Part model, mm, in its own coordinate system. A direction names the side the tool comes from. Round coordinates to 2 decimals unless told otherwise and drop trailing zeros. Order: outer loops, then holes, each group sorted by start corner. A loop starts at its lowest first (then second) coordinate and runs counter-clockwise, first axis right, second up. Notation, with made-up numbers: M 39,34 L 91,34 A19 ccw 91,43 Z; hole C 85,63 d7. An arc over 180 degrees is marked long. One line per question, with ' | ' between items.
from build123d import *

# Parameters (mm, degrees)
BOSS_EXTRUDE1_DEPTH     = 12.7
CUT_EXTRUDE1_REACH      = 14.7
SKETCH2_R               = 0.775
SKETCH4_R               = 12.5
SKETCH4_R_2             = 2.75
BOSS_EXTRUDE3_DEPTH     = 20.5
BOSS_EXTRUDE4_DEPTH     = 20.5
SKETCH5_R               = 1.5
CUT_EXTRUDE2_DEPTH      = 12
CUT_EXTRUDE2_DEPTH_BACK = 2
CUT_EXTRUDE3_DEPTH      = 17


with BuildPart() as part:
    # Sketch1 → Boss-Extrude1 (new body)
    with BuildSketch(Plane(origin=(0, 0, 0), x_dir=(-1, 0, 0), z_dir=(0, 0, -1))):
        Polygon((22.52557458, -1.736588639), (22.52557458, 0.194536921), (19.229808022, 0.93665661), (15.128723263, 11.851737372), (17.063649078, 14.621011813), (15.786423571, 16.069438867), (12.890863827, 14.329165151), (2.313040546, 19.235032954), (1.719665356, 22.560799741), (-0.211460204, 22.560799741), (-0.98374926, 19.271971918), (-11.902473648, 15.180597821), (-14.673902719, 17.112436257), (-16.073066924, 15.781427071), (-14.308800518, 12.900423272), (-19.236913758, 2.332945609), (-22.560976284, 1.730096406), (-22.560976284, -0.201029153), (-19.275488766, -0.987407309), (-15.174404006, -11.902488071), (-17.112216048, -14.669743631), (-15.788139908, -16.075470597), (-12.910837913, -14.305173427), (-2.333014633, -19.21104123), (-1.727718406, -22.534659035), (0.203407153, -22.534659035), (0.978499423, -19.246490729), (11.89722381, -15.155116632), (14.659649692, -17.099807376), (16.072878525, -15.783741196), (14.276312796, -12.922767512), (19.204426036, -2.355289849), align=None)
    extrude(amount=-BOSS_EXTRUDE1_DEPTH)

    # Sketch2 → Cut-Extrude1 (cut, up to next)
    with BuildSketch(Plane(origin=(0, 0, 0), x_dir=(-1, 0, 0), z_dir=(0, 0, -1)), mode=Mode.PRIVATE) as cut_extrude1_sk1:
        with Locations((-0.019773646, -0.00956531)):
            Circle(SKETCH2_R)
    cut_extrude1_tool1 = extrude(cut_extrude1_sk1.sketch, amount=-CUT_EXTRUDE1_REACH, mode=Mode.PRIVATE) & part.part
    add(cut_extrude1_tool1.solids().sort_by_distance((0.019774, -0.009565, 0))[0], mode=Mode.SUBTRACT)

    # Sketch4 → Boss-Extrude3 (add)
    with BuildSketch(Plane(origin=(0, 0, 0), x_dir=(-1, 0, 0), z_dir=(0, 0, -1))):
        Circle(SKETCH4_R)
        Circle(SKETCH4_R_2, mode=Mode.SUBTRACT)
    extrude(amount=BOSS_EXTRUDE3_DEPTH)

    # Sketch4<4> → Boss-Extrude4 (add)
    with BuildSketch(Plane(origin=(0, 0, 0), x_dir=(-1, 0, 0), z_dir=(0, 0, -1))):
        with BuildLine():
            Line((-0.567488363, 2.690809722), (0.726565511, 2.652282518))
            ThreePointArc((0.726565511, 2.652282518), (0.081838079, 2.748782008), (-0.567488363, 2.690809722))
        make_face()
    extrude(amount=BOSS_EXTRUDE4_DEPTH)

    # Sketch5 → Cut-Extrude2 (cut, two sides)
    with BuildSketch(Plane(origin=(0, 4, 0), x_dir=(1, 0, 0), z_dir=(0, 1, 0))) as cut_extrude2_sk:
        with Locations((0, 16.130068411)):
            Circle(SKETCH5_R)
    extrude(amount=CUT_EXTRUDE2_DEPTH, mode=Mode.SUBTRACT)
    extrude(cut_extrude2_sk.sketch, amount=-CUT_EXTRUDE2_DEPTH_BACK, mode=Mode.SUBTRACT)

    # Sketch6 → Cut-Extrude3 (cut)
    with BuildSketch(Plane(origin=(0, 0, -20.5), x_dir=(-1, 0, 0), z_dir=(0, 0, -1))):
        Polygon((4.579538574, 7.537569925), (-4.420461426, 7.805522315), (-4.538346431, 3.845994095), (4.461653569, 3.578041705), align=None)
    extrude(amount=-CUT_EXTRUDE3_DEPTH, mode=Mode.SUBTRACT)


solid = part.part
1) Saw through at A-A (z = -5). List the corners of the cut face in (x, y).
The answers:
outline: C 0,0 d25; hole M -4.58,7.54 L -4.46,3.58 L 4.54,3.85 L 4.42,7.81 Z; hole M -0.73,2.65 A2.75 ccw long 0.57,2.69 Z
2) Which spindle directions (+Z, -Z, +X, -X, +Y, -Y) get a long thin tool onto all of the face, cutting with end or side? Do faces 1 (the face through (6.367, 17.255, 6.261)), 2 (the face through (1.43, 3.04, -16.58)), 3 (the face through (14.37, -15.203, 6.261)), 4 (the face through (-16.083, 13.217, 6.261)), 5 (the face through (0, 6, -3.5)). Say none if no direction does.
The answers:
face 1: +Z, -Z, +Y | face 2: +Y | face 3: +Z, -Z, -Y | face 4: +Z, -Z, -X | face 5: -Z
3) Drop flat-ended pins along their axis: pin 1 (2.5 mm diameter, centred on x = 0, z = -16.13, fed in from +Y); pin 2 (1.8 mm diameter, centred on x = 0.02, y = -0.01, fed in from +Z); pin 3 (8 mm diameter, centred on y = -10.5, z = 7.5, fed in from -X); pin 4 (5 mm diameter, centred on y = -15, z = 4.5, fed in from -X). Give the stop position or say it passes through.
The answers:
pin 1: stops at y = -2.45 | pin 2: stops at z = 12.7 | pin 3: stops at x = -17.27 | pin 4: stops at x = -16.07
4) Probe line 1 (Z direction, x = 0, y = 3); line 2 (Z direction, x = 1, y = -2.5); line 3 (X direction, y = 10, z = -16). List the from-to ranges inside material, lowest first. Write a range as [from, to].
The answers:
line 1: z = [-20.5, -17.63], [-14.63, 12.7] | line 2: z = [0, 12.7] | line 3: x = [-7.5, -1.49], [1.49, 7.5]
5) Saw through at C-C (x = -7). List the corners of the cut face in (y, z), plus the area to 3 significant figures.
The answers:
outline: M -16.99,0 L -10.36,0 L -10.36,-20.5 L 10.36,-20.5 L 10.36,0 L 17.06,0 L 17.06,12.7 L -16.99,12.7 Z | area: 857 mm²
6) Two-plate mould, pull along Y, no slides. Class faces 6 (the face through (-13.259, -16.114, 6.261)), 7 (the face through (-1, 1, 0)), 8 (the face through (-7.676, 16.748, 6.261)): released by +Y, released by -Y, zero draft, split by the parting line, or undercut.
The answers:
face 6: released by -Y | face 7: undercut | face 8: released by +Y
7) Saw through at B-B (x = 8.5). List the corners of the cut face in (y, z), plus the area to 3 significant figures.
The answers:
outline: M -16.35,0 L -9.17,0 L -9.17,-20.5 L 9.17,-20.5 L 9.17,0 L 16.46,0 L 16.46,12.7 L -16.35,12.7 Z | area: 792 mm²
